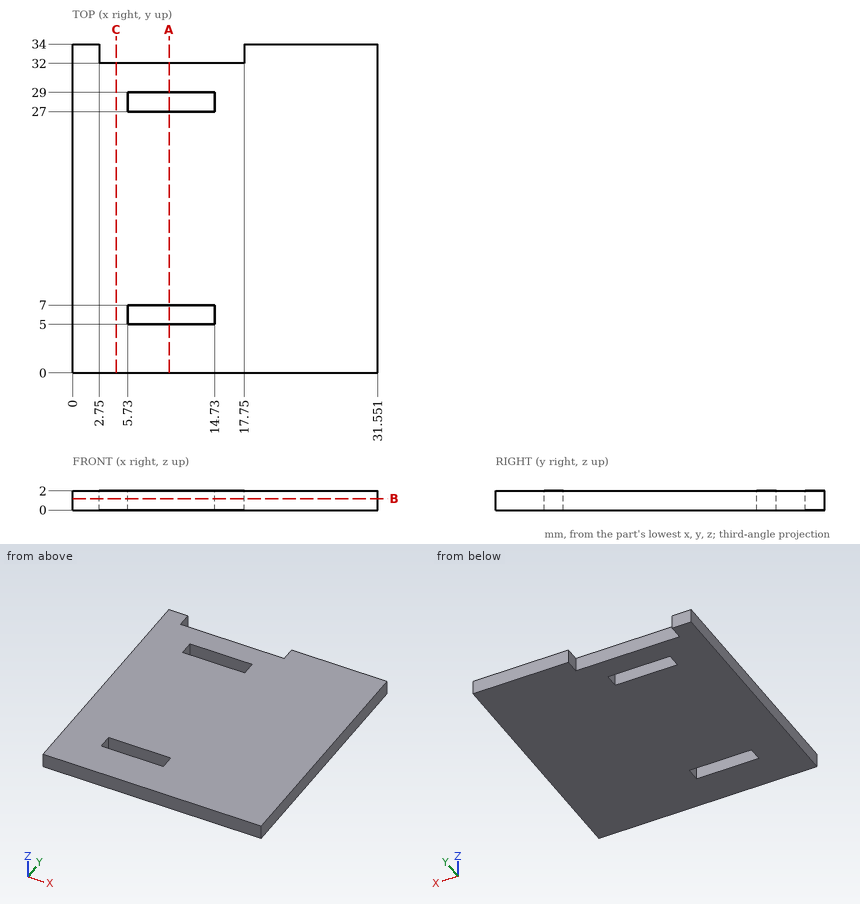
Study the drawing (mm; zero at the part's minimum x, y, z) and answer. Round coordinates to 2 decimals unless told otherwise and drop trailing zeros. Loops run counter-clockwise (first coordinate to the right, second up) from the corner with the lowest first, then second, coordinate; pieces in that order, holes last.
Q1. Given pin 1 Ø1 at (y, z) = (33.5, 1) entering from -X; pin 2 Ø1 at (x, z) = (9, 1.5) entering from +Y, each flat-ended and moving along its own axis, determine where each tip first touches the part or whether it passes through.
Q2. Section A-A, the plane x = 10 is taken. Determine the outline of the cut face in (y, z), then the cut area to 3 significant figures.
Q3. Section C-C, the plane x = 4.5 is taken. Determine the outline of the cut face in (y, z), then the cut area to 3 significant figures.
Q4. Section B-B, the plane z = 1.2 is taken. Determine the outline of the cut face in (x, y), then the cut area to 3 significant figures.
Q5. Find the intervals of material crossed by line 1 (Y direction, x = 14, z = 0.2); line 2 (X direction, y = 28.5, z = 1.6); line 3 (Y direction, x = 4, z = 1.9), in increasing order.
Completed:
1. pin 1: stops at x = 0
1. pin 2: stops at y = 32
2. outline: (0, 0) - (5, 0) - (5, 2) - (0, 2) - close; (7, 0) - (27, 0) - (27, 2) - (7, 2) - close; (29, 0) - (32, 0) - (32, 2) - (29, 2) - close
2. area: 56.0 mm2
3. outline: (0, 0) - (32, 0) - (32, 2) - (0, 2) - close
3. area: 64.0 mm2
4. outline: (0, 0) - (31.55, 0) - (31.55, 34) - (17.75, 34) - (17.75, 32) - (2.75, 32) - (2.75, 34) - (0, 34) - close; hole (5.73, 5) - (14.73, 5) - (14.73, 7) - (5.73, 7) - close; hole (5.73, 27) - (14.73, 27) - (14.73, 29) - (5.73, 29) - close
4. area: 1,010 mm2
5. line 1: y = 0 to 5, 7 to 27, 29 to 32
5. line 2: x = 0 to 5.73, 14.73 to 31.55
5. line 3: y = 0 to 32
